Job drawing, mm, ordinate dimensions from the low corner. One solid piece. Give positions to 0.01 mm unless a question says otherwise; leave off trailing zeros. Loops run counter-clockwise (first coordinate to the right, second up) from the corner with the lowest first, then second, coordinate; pieces in that order, holes last. Notation, with made-up numbers: (23, 87) -> (79, 87) arc R11 ccw to (79, 91) -> close; hole circle Ø2 at (-3, 53). An arc over 180 degrees is marked (long way). Use one line per item in the form item = value.
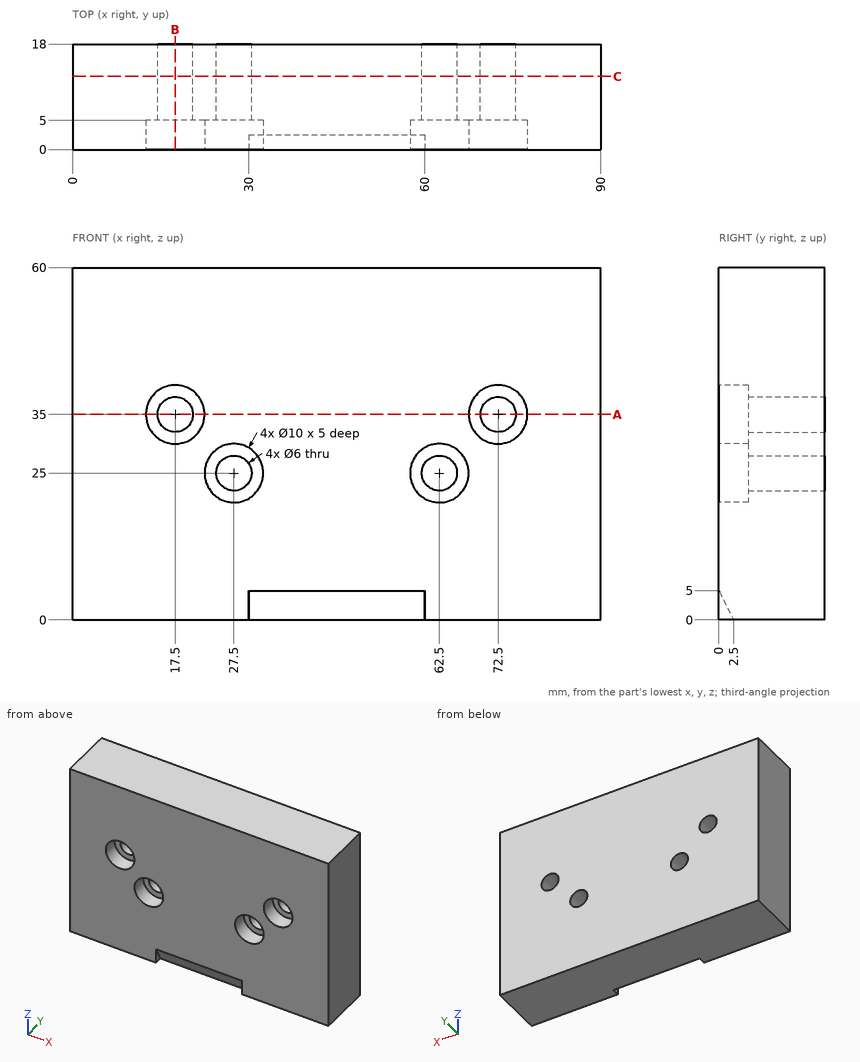
1. Cut at B-B, the plane x = 17.5. Write the cut outline in (y, z).
Result sheet:
outline = (0, 0) -> (18, 0) -> (18, 32) -> (5, 32) -> (5, 30) -> (0, 30) -> close; (0, 40) -> (5, 40) -> (5, 38) -> (18, 38) -> (18, 60) -> (0, 60) -> close
2. Cut at A-A, the plane z = 35. Write the cut outline in (x, y), then the cut area to 3 significant figures.
Result sheet:
outline = (0, 0) -> (12.5, 0) -> (12.5, 5) -> (14.5, 5) -> (14.5, 18) -> (0, 18) -> close; (20.5, 5) -> (22.5, 5) -> (22.5, 0) -> (67.5, 0) -> (67.5, 5) -> (69.5, 5) -> (69.5, 18) -> (20.5, 18) -> close; (75.5, 5) -> (77.5, 5) -> (77.5, 0) -> (90, 0) -> (90, 18) -> (75.5, 18) -> close
area = 1,360 mm^2
3. Drop flat-ended pins along their axis: P1, Ø9.5, axis at x = 27.5, z = 25, coming from the -Y side; P2, Ø3.5, axis at x = 62.5, z = 25, coming from the -Y side. Give the stop position or say it passes through.
Result sheet:
P1 = 5
P2 = through
4. Drill centre lines: line 1 (Z direction, x = 62.5, y = 15.25); line 2 (Z direction, x = 17.5, y = 2). Where is each one in solid material? Low to high.
Result sheet:
line_1 = 0 to 22, 28 to 60
line_2 = 0 to 30, 40 to 60
5. Cut at C-C, the plane y = 12.5. Write the cut outline in (x, z), then the cut area to 3 significant figures.
Result sheet:
outline = (0, 0) -> (90, 0) -> (90, 60) -> (0, 60) -> close; hole circle Ø6 at (17.5, 35); hole circle Ø6 at (27.5, 25); hole circle Ø6 at (62.5, 25); hole circle Ø6 at (72.5, 35)
area = 5,290 mm^2
